Build history of the part. All positions in model axes, mm. Face numbers are marked on the shaded views. A direction names the side the tool comes from. Round coordinates to 2 decimals unless told otherwise and drop trailing zeros. Write each loop counter-clockwise with the first axis right and the second up, starting at its lowest first coordinate (ties: lowest second). Pieces come first, ordered by that corner, then holes. Notation, with made-up numbers: (-23, 60.25) -> (9, 60.25) arc R18 ccw to (9, 77.25) -> close; hole circle Ø4 at (21, 48). An arc over 180 degrees is marked (long way). Answer in a Markdown table with one row per item.
```python
from build123d import *

# Parameters (mm, degrees)
BOSS_EXTRUDE1_DEPTH            = 100
SKETCH2_R                      = 14
BOSS_EXTRUDE2_DEPTH            = 20
SKETCH3_R                      = 12
BOSS_EXTRUDE3_DEPTH            = 8
FILLET1_R                      = 4
SKETCH4_R                      = 4
BOSS_EXTRUDE4_DEPTH            = 10
FILLET2_R                      = 2
SKETCH6_R                      = 14
BOSS_EXTRUDE6_DEPTH            = 20
SKETCH7_R                      = 11
SKETCH7_R_2                    = 10
BOSS_EXTRUDE7_DEPTH            = 20
CUT_EXTRUDE1_REACH             = 17.529
CUT_EXTRUDE1_DIRECTION_2_REACH = 17.529
CUT_EXTRUDE2_REACH             = 17.529
CUT_EXTRUDE2_DIRECTION_2_REACH = 17.529
SKETCH10_R                     = 10
BOSS_EXTRUDE8_DEPTH            = 8
SKETCH11_R                     = 3
BOSS_EXTRUDE9_DEPTH            = 6
FILLET3_R                      = 3


with BuildPart() as part:
    # Sketch1 → Boss-Extrude1 (new body)
    with BuildSketch(Plane.XY):
        Polygon((-15.529142706, 0), (-13.448632083, -7.764571353), (-7.764571353, -13.448632083), (0, -15.529142706), (7.764571353, -13.448632083), (13.448632083, -7.764571353), (15.529142706, 0), (13.448632083, 7.764571353), (7.764571353, 13.448632083), (0, 15.529142706), (-7.764571353, 13.448632083), (-13.448632083, 7.764571353), align=None)
    extrude(amount=-BOSS_EXTRUDE1_DEPTH)

    # Sketch2 → Boss-Extrude2 (add)
    with BuildSketch(Plane.XY):
        Circle(SKETCH2_R)
    extrude(amount=BOSS_EXTRUDE2_DEPTH)

    # Sketch3 → Boss-Extrude3 (add)
    with BuildSketch(Plane.XY.offset(20)):
        Circle(SKETCH3_R)
    extrude(amount=BOSS_EXTRUDE3_DEPTH)

    # Fillet1
    fillet1_edges = [part.edges().sort_by_distance(p)[0] for p in [
        (-12, 0, 28),
    ]]
    fillet(fillet1_edges, radius=FILLET1_R)

    # Sketch4 → Boss-Extrude4 (add)
    with BuildSketch(Plane.XY.offset(28)):
        Circle(SKETCH4_R)
    extrude(amount=BOSS_EXTRUDE4_DEPTH)

    # Fillet2
    fillet2_edges = [part.edges().sort_by_distance(p)[0] for p in [
        (-4, 0, 38),
    ]]
    fillet(fillet2_edges, radius=FILLET2_R)

    # Sketch6 → Boss-Extrude6 (add)
    with BuildSketch(Plane(origin=(0, 0, -100), x_dir=(-1, 0, 0), z_dir=(0, 0, -1))):
        Circle(SKETCH6_R)
    extrude(amount=BOSS_EXTRUDE6_DEPTH)

    # Sketch7 → Boss-Extrude7 (add)
    with BuildSketch(Plane(origin=(0, 0, -120), x_dir=(-1, 0, 0), z_dir=(0, 0, -1))):
        Circle(SKETCH7_R)
        Circle(SKETCH7_R_2, mode=Mode.SUBTRACT)
    extrude(amount=BOSS_EXTRUDE7_DEPTH)

    # Sketch8 → Cut-Extrude1 (cut, up to next)
    with BuildSketch(Plane(origin=(0, 0, 0), x_dir=(0, 0, -1), z_dir=(1, 0, 0)), mode=Mode.PRIVATE) as cut_extrude1_sk1:
        with BuildLine():
            Line((145, -5), (135, -5))
            ThreePointArc((135, -5), (130, 0), (135, 5))
            Line((135, 5), (145, 5))
            Line((145, 5), (145, -5))
        make_face()
    cut_extrude1_tool1 = extrude(cut_extrude1_sk1.sketch, amount=-CUT_EXTRUDE1_REACH, mode=Mode.PRIVATE) & part.part
    add(cut_extrude1_tool1.solids().sort_by_distance((0, 0, -137.991792))[0], mode=Mode.SUBTRACT)

    # Sketch8 → Cut-Extrude1 direction 2 (cut, up to next)
    with BuildSketch(Plane(origin=(0, 0, 0), x_dir=(0, 0, -1), z_dir=(1, 0, 0)), mode=Mode.PRIVATE) as cut_extrude1_direction_2_sk1:
        with BuildLine():
            Line((145, -5), (135, -5))
            ThreePointArc((135, -5), (130, 0), (135, 5))
            Line((135, 5), (145, 5))
            Line((145, 5), (145, -5))
        make_face()
    cut_extrude1_direction_2_tool1 = extrude(cut_extrude1_direction_2_sk1.sketch, amount=CUT_EXTRUDE1_DIRECTION_2_REACH, mode=Mode.PRIVATE) & part.part
    add(cut_extrude1_direction_2_tool1.solids().sort_by_distance((0, 0, -137.991792))[0], mode=Mode.SUBTRACT)

    # Sketch9 → Cut-Extrude2 (cut, up to next)
    with BuildSketch(Plane(origin=(0, 0, 0), x_dir=(1, 0, 0), z_dir=(0, 1, 0)), mode=Mode.PRIVATE) as cut_extrude2_sk1:
        with BuildLine():
            Line((-5, 132.755823636), (-5, 147.244176364))
            Line((-5, 147.244176364), (5, 147.244176364))
            Line((5, 147.244176364), (5, 132.755823636))
            ThreePointArc((5, 132.755823636), (0, 127.755823636), (-5, 132.755823636))
        make_face()
    cut_extrude2_tool1 = extrude(cut_extrude2_sk1.sketch, amount=-CUT_EXTRUDE2_REACH, mode=Mode.PRIVATE) & part.part
    add(cut_extrude2_tool1.solids().sort_by_distance((0, 0, -138.00269))[0], mode=Mode.SUBTRACT)

    # Sketch9 → Cut-Extrude2 direction 2 (cut, up to next)
    with BuildSketch(Plane(origin=(0, 0, 0), x_dir=(1, 0, 0), z_dir=(0, 1, 0)), mode=Mode.PRIVATE) as cut_extrude2_direction_2_sk1:
        with BuildLine():
            Line((-5, 132.755823636), (-5, 147.244176364))
            Line((-5, 147.244176364), (5, 147.244176364))
            Line((5, 147.244176364), (5, 132.755823636))
            ThreePointArc((5, 132.755823636), (0, 127.755823636), (-5, 132.755823636))
        make_face()
    cut_extrude2_direction_2_tool1 = extrude(cut_extrude2_direction_2_sk1.sketch, amount=CUT_EXTRUDE2_DIRECTION_2_REACH, mode=Mode.PRIVATE) & part.part
    add(cut_extrude2_direction_2_tool1.solids().sort_by_distance((0, 0, -138.00269))[0], mode=Mode.SUBTRACT)

    # Sketch10 → Boss-Extrude8 (add)
    with BuildSketch(Plane(origin=(0, 0, -120), x_dir=(-1, 0, 0), z_dir=(0, 0, -1))):
        Circle(SKETCH10_R)
    extrude(amount=BOSS_EXTRUDE8_DEPTH)

    # Sketch11 → Boss-Extrude9 (add)
    with BuildSketch(Plane(origin=(0, 0, -128), x_dir=(-1, 0, 0), z_dir=(0, 0, -1))):
        Circle(SKETCH11_R)
    extrude(amount=BOSS_EXTRUDE9_DEPTH)

    # Fillet3
    fillet3_edges = [part.edges().sort_by_distance(p)[0] for p in [
        (3, 0, -134),
    ]]
    fillet(fillet3_edges, radius=FILLET3_R)


solid = part.part
```
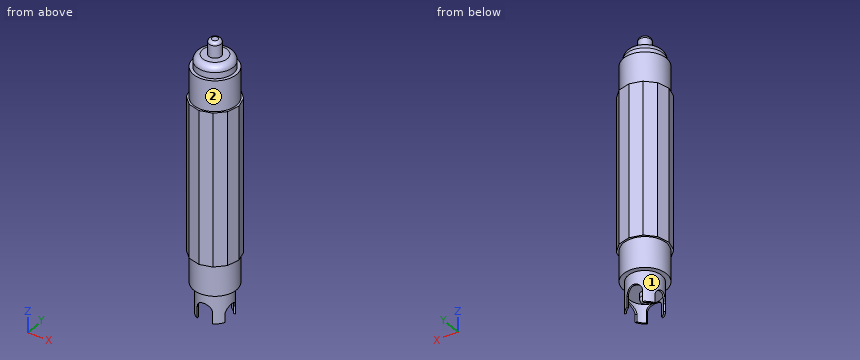
Q1. Saw through at A-A on z = -68.5. Write the cut outline in (x, y).
A:
| item | result |
|---|---|
| outline | (-15.53, 0) -> (-13.45, -7.76) -> (-7.76, -13.45) -> (0, -15.53) -> (7.76, -13.45) -> (13.45, -7.76) -> (15.53, 0) -> (13.45, 7.76) -> (7.76, 13.45) -> (0, 15.53) -> (-7.76, 13.45) -> (-13.45, 7.76) -> close |
Q2. Wall check: line 1 (Z direction, x = -7.5, y = -4); line 2 (X direction, y = -11.5, z = 9); line 3 (Z direction, x = 10, y = 7). Give the ranges that are in metal, low to high. Write a range as [from, to].
A:
| item | result |
|---|---|
| line 1 | [-128, 27.97] |
| line 2 | [-7.98, 7.98] |
| line 3 | [-120, 20] |
Q3. Drop flat-ended pins along their axis: P1, Ø0.9, axis at x = -9.5, z = -136.5, coming from the -Y side; P2, Ø1, axis at x = 9.5, z = -8.5, coming from the +Y side; P3, Ø1, axis at x = -4, y = -6, coming from the -Z side. Give the stop position or say it passes through.
A:
| item | result |
|---|---|
| P1 | y = -6.25 |
| P2 | y = 12.21 |
| P3 | z = -128 |
Q4. Which spindle directions (+Z, -Z, +X, -X, +Y, -Y) get a long thin tool onto all of the face, cutting with end or side? Do the marked faces 1 and 2. Say none if no direction does.
A:
| item | result |
|---|---|
| face 1 | -Z |
| face 2 | +Z |
